from build123d import *

# Parameters (mm, degrees)
F0_W      = 1100
F0_H      = 500
F1_DEPTH  = 20
F4_DEPTH  = 20
F5_W      = 20
F5_H      = 500
F6_DEPTH  = 460
F9_DEPTH  = 20
F10_W     = 775
F10_H     = 20
F11_DEPTH = 425
F12_W     = 1100
F12_H     = 20
F13_DEPTH = 300
F14_W     = 20
F14_H     = 230
F15_DEPTH = 300
F16_W     = 20
F16_H     = 250
F17_DEPTH = 295
F19_DEPTH = 20
F20_DEPTH = 20


with BuildPart() as f1:
    # F0 (on Top) → F1 (new body)
    with BuildSketch(Plane.XY):
        Rectangle(F0_W, F0_H)
    extrude(amount=F1_DEPTH)

    # F3 (on offset) → F4 (join)
    with BuildSketch(Plane.YZ.offset(550)):
        Polygon((250, -465), (250, 0), (250, 25), (-150, 25), (-150, -465), align=None)
    extrude(amount=F4_DEPTH)

    # F5 (on face) → F6 (join)
    with BuildSketch(Plane.XY):
        with Locations((-380, 0)):
            Rectangle(F5_W, F5_H)
    extrude(amount=-F6_DEPTH)

    # F8 (on offset) → F9 (join)
    with BuildSketch(Plane(origin=(0, 155, 0), x_dir=(-1, 0, 0), z_dir=(0, 1, 0))):
        Polygon((370, 0), (0, 0), (-420, 0), (-420, -460), (370, -460), align=None)
    extrude(amount=-F9_DEPTH)

    # F10 (on face) → F11 (join)
    with BuildSketch(Plane.XZ.offset(-135)):
        with Locations((162.5, -210)):
            Rectangle(F10_W, F10_H)
    extrude(amount=F11_DEPTH)

    # F12 (on face) → F13 (join)
    with BuildSketch(Plane.XY.offset(20)):
        with Locations((0, 240)):
            Rectangle(F12_W, F12_H)
    extrude(amount=F13_DEPTH)

    # F14 (on face) → F15 (join)
    with BuildSketch(Plane.XY.offset(20)):
        with Locations((-540, 115)):
            Rectangle(F14_W, F14_H)
    extrude(amount=F15_DEPTH)

    # F16 (on face) → F17 (join)
    with BuildSketch(Plane.XY.offset(25)):
        with Locations((560, 125)):
            Rectangle(F16_W, F16_H)
    extrude(amount=F17_DEPTH)

    # F18 (on face) → F19 (join)
    with BuildSketch(Plane.XY.offset(320)):
        Polygon((-300, 250), (-550, 250), (-550, 0), (-300, 0), (-300, 150), (320, 150), (320, 0), (570, 0), (570, 250), (320, 250), align=None)
    extrude(amount=F19_DEPTH)

    # F18 (on face) → F20 (join)
    with BuildSketch(Plane.XY.offset(320)):
        Polygon((-300, 250), (-550, 250), (-550, 0), (-300, 0), (-300, 150), (320, 150), (320, 0), (570, 0), (570, 250), (320, 250), align=None)
    extrude(amount=F20_DEPTH)


solid = f1.part
Here's how the part is built. I have some questions about the finished solid (model axes, mm). A direction names the side the tool comes from. Round coordinates to 2 decimals unless told otherwise and drop trailing zeros. Loops run counter-clockwise (first coordinate to the right, second up) from the corner with the lowest first, then second, coordinate; pieces in that order, holes last. Notation, with made-up numbers: (-29.5, -31) - (8.5, -31) arc R23 ccw to (8.5, 7) - close; hole circle Ø6 at (-38.75, 89.5). An arc over 180 degrees is marked (long way). One line per question, with ' | ' between items. Start each with the question number.
Q1. I want a section at D-D (y = -207.5). Write out the boundary of the cut face in (x, z), then the cut area to 3 significant figures.
Q2. Please list where these lines run through material, in increasing order: line 1 (Z direction, x = 403, y = -222.5); line 2 (Z direction, x = -117, y = 208); line 3 (Z direction, x = 386, y = 21). Write a range as [from, to].
Q3. Will these pins go through, and if not, where does the flat tip stop? pin 1 (4 mm diameter, centred on y = -70, z = 28.5, fed in from +X); pin 2 (6 mm diameter, centred on x = 44.5, z = 333, fed in from -Y); pin 3 (6 mm diameter, centred on x = 184.5, y = -120, fed in from +Z); pin 4 (1 mm diameter, centred on y = 161.5, z = -274.5, fed in from -X).
Q4. I want a section at A-A (z = -181). Write out the boundary of the cut face in (x, y), then the cut area to 3 significant figures.
Q5. We'd pull the mould along Z, two halves only. Please class faces 4 (the flat face through (-537, 0, 250)), 5 (the flat face through (157, -75, -220)), 6 (the flat face through (-530, 113, 168)): +Z half, -Z half, draft (parallel to the pull), parting line (faces both ways), or undercut.
Q6. I want a section at B-B (y = 201). Write out the boundary of the cut face in (x, z).
Q7. For faces 1 (the flat face through (-167, 149, -460)), 2 (the flat face through (556, 0, 252)), 3 (the flat face through (-8, -7, 20)), which set-ups out of +Z, -Z, +X, -X, +Y, -Y let a thin tool reach every point of the face, with its end or its side?
Q8. I want a section at C-C (x = 353). Write out the boundary of the cut face in (y, z).
Response values:
1) outline: (-550, 0) - (-390, 0) - (-390, -460) - (-370, -460) - (-370, 0) - (550, 0) - (550, 20) - (-550, 20) - close; (-225, -220) - (550, -220) - (550, -200) - (-225, -200) - close | area: 46,700 mm²
2) line 1: z = [-220, -200], [0, 20] | line 2: z = [0, 20], [320, 340] | line 3: z = [-220, -200], [0, 20], [320, 340]
3) pin 1: passes through | pin 2: stops at y = 150 | pin 3: stops at z = 20 | pin 4: stops at x = -390
4) outline: (-390, -250) - (-370, -250) - (-370, 135) - (420, 135) - (420, 155) - (-370, 155) - (-370, 250) - (-390, 250) - close; (550, -150) - (570, -150) - (570, 250) - (550, 250) - close | area: 33,800 mm²
5) face 4: draft | face 5: -Z half | face 6: undercut
6) outline: (-550, 0) - (-390, 0) - (-390, -460) - (-370, -460) - (-370, 0) - (550, 0) - (550, -465) - (570, -465) - (570, 340) - (-550, 340) - close; hole (-530, 20) - (550, 20) - (550, 320) - (-530, 320) - close
7) face 1: -Z, -X, +Y, -Y | face 2: +Z, +X, -X, -Y | face 3: -Y
8) outline: (-290, -220) - (135, -220) - (135, -460) - (155, -460) - (155, 0) - (250, 0) - (250, 340) - (0, 340) - (0, 320) - (230, 320) - (230, 20) - (-250, 20) - (-250, 0) - (135, 0) - (135, -200) - (-290, -200) - close
